The model under review builds one solid part; all positions refer to its coordinate system, in mm. A direction names the side the tool comes from. Give positions to 0.01 mm unless a question says otherwise; leave off trailing zeros. Order: outer loops, then holes, each group sorted by start corner. A loop starts at its lowest first (then second) coordinate and runs counter-clockwise, first axis right, second up. Notation, with made-up numbers: (32.5, 1) -> (62.5, 1) arc R28 ccw to (62.5, 30) -> close; hole circle Ø3 at (35, 44.25). An arc over 180 degrees is marked (long way). Answer as a JSON object with one key per item and string values. Group by question number.
from build123d import *

# Parameters (mm, degrees)
SKETCH061_W                    = 10
SKETCH061_H                    = 5
PAD017_DEPTH                   = 1.7
SKETCH062_W                    = 3.516788
SKETCH062_H                    = 1.8
PAD018_DEPTH                   = 4
PART_MIRRORING_PLACEMENT_ANGLE = 180


with BuildPart() as obj1:
    # Sketch061 → Pad017 (new body)
    with BuildSketch(Plane.XY):
        Polygon((30, 0), (51, 0), (51, 9), (31.917717, 9), (31.217717, 9.7), (30.7, 9.7), (30, 9), (30, 7), (37, 7), (37, 2), (30, 2), align=None)
        with Locations((44, 4.5)):
            Rectangle(SKETCH061_W, SKETCH061_H, mode=Mode.SUBTRACT)
    extrude(amount=PAD017_DEPTH)

    # Sketch062 → Pad018 (join)
    with BuildSketch(Plane.XY):
        with Locations((31.758394, 6.923936)):
            Rectangle(SKETCH062_W, SKETCH062_H)
    extrude(amount=PAD018_DEPTH)


with BuildPart() as obj1_petg:
    # Part__Mirroring: instance of obj1
    add(obj1.part.mirror(Plane(origin=(0, 0, 0), x_dir=(0, 1, 0), z_dir=(0, 0, 1))))


with BuildPart() as obj1_petg_1:
    # Part__Mirroring placement: moved
    add(obj1_petg.part.moved(Location((0, -1, 0))).rotate(Axis((0, -1, 0), (1, 0, 0)), PART_MIRRORING_PLACEMENT_ANGLE))


solid = obj1_petg_1.part
1. For probe 1 along X at (y, z) = (-5.25, 1.35); probe 2 along X at (y, z) = (-7.5, 2.9); probe 3 along Y at (x, z) = (35.25, 1.05), list the stretches that pass through material, from the lowest coordinate up. Write a range as [from, to].
2. Take a section at D-D on x = 36.25. Give the boundary of the cut face in (y, z), plus the area to 3 significant figures.
3. Take a section at A-A on x = 32.25. Give the boundary of the cut face in (y, z), plus the area to 3 significant figures.
4. Take a section at C-C on y = -4.75. Give the boundary of the cut face in (x, z), plus the area to 3 significant figures.
5. Machinability: for faces 4 (the flat face through (35, -8, 1)), 5 (the flat face through (34, -3, 1)), 6 (the flat face through (32, -8.824, 3)), which of the approach directions +Z, -Z, +X, -X, +Y, -Y give a long, thin tool a straight path to every point of the face, cutting with its end or side? Answer none if there is none.
6. For pin 1 (2 mm diameter, centred on y = -5, z = 3.5, fed in from +X); pin 2 (1.4 mm diameter, centred on y = -6.5, z = 1, fed in from -X); pin 3 (1.9 mm diameter, centred on x = 45.5, z = 0.5, fed in from -Y); pin 4 (1.4 mm diameter, centred on y = -6, z = 0.5, fed in from -X), all flat-tipped, find the tip position at first contact; note any pin that passes through.
7. Draft analysis for pull direction X (two halves, no side actions). For faces 1 (the flat face through (44, -8, 1)), 2 (the flat face through (40, -1, 1)), 3 (the flat face through (51, -5, 1)), state which applies: pulls with the +X half, pulls with the -X half, needs draft (parallel to the pull), parting line crosses it, or undercut.
8. Take a section at B-B on z = 1.45. Give the boundary of the cut face in (x, y).
Checks:
{
 "1": {"probe 1": "x = [37, 39], [49, 51]", "probe 2": "x = [30, 33.52]", "probe 3": "y = [-10, -8], [-3, -1]"},
 "2": {"outline": "(-10, 0) -> (-8, 0) -> (-8, 1.7) -> (-10, 1.7) -> close; (-3, 0) -> (-1, 0) -> (-1, 1.7) -> (-3, 1.7) -> close", "area": "6.80 mm2"},
 "3": {"outline": "(-10, 0) -> (-7.02, 0) -> (-7.02, 4) -> (-8.82, 4) -> (-8.82, 1.7) -> (-10, 1.7) -> close; (-3, 0) -> (-1, 0) -> (-1, 1.7) -> (-3, 1.7) -> close", "area": "12.6 mm2"},
 "4": {"outline": "(37, 0) -> (39, 0) -> (39, 1.7) -> (37, 1.7) -> close; (49, 0) -> (51, 0) -> (51, 1.7) -> (49, 1.7) -> close", "area": "6.80 mm2"},
 "5": {"face 4": "+Z, -Z", "face 5": "+Z, -Z, -X", "face 6": "+Z, +X, -X, -Y"},
 "6": {"pin 1": "passes through", "pin 2": "stops at x = 30", "pin 3": "stops at y = -10", "pin 4": "stops at x = 37"},
 "7": {"face 1": "undercut", "face 2": "needs draft", "face 3": "pulls with the +X half"},
 "8": {"outline": "(30, -10) -> (30.7, -10.7) -> (31.22, -10.7) -> (31.92, -10) -> (51, -10) -> (51, -1) -> (30, -1) -> (30, -3) -> (37, -3) -> (37, -8) -> (33.52, -8) -> (33.52, -7.02) -> (30, -7.02) -> close; hole (39, -8) -> (49, -8) -> (49, -3) -> (39, -3) -> close"}
}
